from build123d import *

# Parameters (mm, degrees)
SKETCH2_W           = 12.7
SKETCH2_H           = 12.7
BOSS_EXTRUDE1_DEPTH = 6.35
SKETCH3_R           = 3.175
BOSS_EXTRUDE2_DEPTH = 12.7


with BuildPart() as part:
    # Sketch2 → Boss-Extrude1 (new body)
    with BuildSketch(Plane.XY):
        with Locations((6.35, 6.35)):
            Rectangle(SKETCH2_W, SKETCH2_H)
    extrude(amount=BOSS_EXTRUDE1_DEPTH)

    # Sketch3 → Boss-Extrude2 (add)
    with BuildSketch(Plane.XY.offset(6.35)):
        with Locations((6.35, 6.35)):
            Circle(SKETCH3_R)
    extrude(amount=BOSS_EXTRUDE2_DEPTH)


solid = part.part
Work out the finished part from the listing and answer in its coordinate system (mm). A direction names the side the tool comes from. Give positions to 0.01 mm unless a question says otherwise; leave off trailing zeros. Order: outer loops, then holes, each group sorted by start corner. A loop starts at its lowest first (then second) coordinate and runs counter-clockwise, first axis right, second up. Notation, with made-up numbers: M -27.75,-2 L 26.25,-2 A26 ccw 26.25,15 Z; hole C 69.25,67.5 d7. An arc over 180 degrees is marked long. Return JSON: item names as keys, results as strings.
Q1. Find the intervals of material crossed by line 1 along Z through (x, y) = (12, 7.5); line 2 along Y through (x, z) = (4.5, 15.5); line 3 along X through (y, z) = (5, 14.5), in increasing order. Write a range as [from, to].
Answer below:
{"line 1": "z = [0, 6.35]", "line 2": "y = [3.77, 8.93]", "line 3": "x = [3.48, 9.22]"}
Q2. Which of the six approach directions +Z, -Z, +X, -X, +Y, -Y give full straight-line access (tool end or side, diameter ignored) to faces 1 (the face through (12.7, 6, 3)), 2 (the face through (4.01, 8.496, 12.611))?
Answer below:
{"face 1": "+Z, -Z, +X, +Y, -Y", "face 2": "+Z"}
Q3. Find section A-A, the plane y = 6.35. Write down the section's boundary in (x, z) (3 decimals).
Answer below:
{"outline": "M 0,0 L 12.7,0 L 12.7,6.35 L 9.525,6.35 L 9.525,19.05 L 3.175,19.05 L 3.175,6.35 L 0,6.35 Z"}
Q4. Find section D-D, the plane x = 1.5. Write down the section's boundary in (y, z), and give its area (3 significant figures).
Answer below:
{"outline": "M 0,0 L 12.7,0 L 12.7,6.35 L 0,6.35 Z", "area": "80.6 mm^2"}
Q5. Find section C-C, the plane z = 12.75. Write down the section's boundary in (x, y) (3 decimals).
Answer below:
{"outline": "C 6.35,6.35 d6.35"}
Q6. Each of these flat-tipped pins is pushed along its axis until it touches: pin 1 (6 mm diameter, centred on x = 2, y = 9, fed in from -Z); pin 2 (2 mm diameter, centred on x = 9.5, z = 12, fed in from -Y); pin 3 (5 mm diameter, centred on y = 3.5, z = 15.5, fed in from -X). Where does it stop, or does it pass through?
Answer below:
{"pin 1": "stops at z = 0", "pin 2": "stops at y = 4.01", "pin 3": "stops at x = 3.19"}
